Here's how the part is built. I have some questions about the finished solid (model axes, mm). Face numbers are marked on the shaded views. A direction names the side the tool comes from. Round coordinates to 2 decimals unless told otherwise and drop trailing zeros. Order: outer loops, then holes, each group sorted by start corner. A loop starts at its lowest first (then second) coordinate and runs counter-clockwise, first axis right, second up.
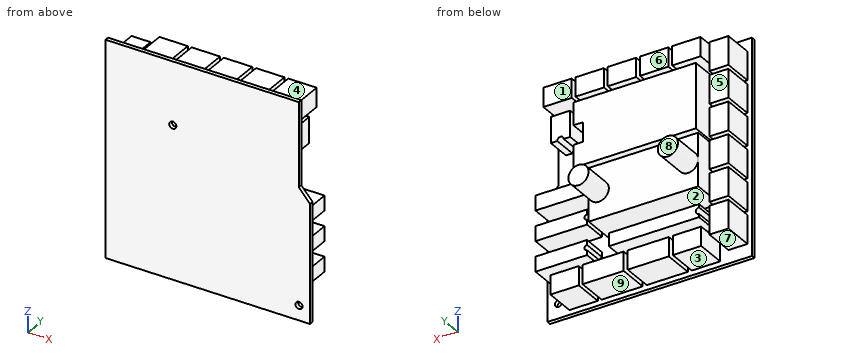
```python
from build123d import *

# Parameters (mm, degrees)
BOSS_EXTRUDE1_DEPTH = 1.5875
SKETCH2_R           = 1.3999972
CUT_EXTRUDE1_DEPTH  = 117.995510328
BOSS_EXTRUDE2_DEPTH = 11.90625
SKETCH4_W           = 43.17991364
SKETCH4_H           = 20.827958344
BOSS_EXTRUDE3_DEPTH = 13.49375
SKETCH6_R           = 3.96875
BOSS_EXTRUDE4_DEPTH = 12.7
BOSS_EXTRUDE5_DEPTH = 9.525


with BuildPart() as part:
    # Sketch1 → Boss-Extrude1 (new body)
    with BuildSketch(Plane(origin=(0, 0, 0), x_dir=(1, 0, 0), z_dir=(0, 1, 0))):
        Polygon((0.038099924, 84.724030552), (0.038099924, 0), (76.258247483, 0), (76.258247483, 33.070733858), (80.667638664, 38.11002378), (80.667638664, 84.724030552), align=None)
    extrude(amount=BOSS_EXTRUDE1_DEPTH)

    # Sketch2 → Cut-Extrude1 (cut, through all)
    with BuildSketch(Plane(origin=(0, 1.5875, 0), x_dir=(1, 0, 0), z_dir=(0, 1, 0))):
        with Locations(Location((76.336947326, 78.897342205, 0), (0, 0, 270))):
            Circle(SKETCH2_R)
        with Locations(Location((26.573446853, 24.724250551, 0), (0, 0, 270))):
            Circle(SKETCH2_R)
    extrude(amount=-CUT_EXTRUDE1_DEPTH, mode=Mode.SUBTRACT)

    # Sketch3 → Boss-Extrude2 (add)
    with BuildSketch(Plane(origin=(0, 1.5875, 0), x_dir=(1, 0, 0), z_dir=(0, 1, 0))):
        Polygon((60.822778354, 75.352649294), (60.822778354, 81.852636294), (60.822778354, 82.852634294), (72.022755954, 82.852634294), (72.022755954, 81.852636294), (72.022755954, 75.352649294), align=None)
        Polygon((59.322781354, 82.852634294), (59.322781354, 81.852636294), (59.322781354, 75.352649294), (43.122813754, 75.352649294), (43.122813754, 81.852636294), (43.122813754, 82.852634294), align=None)
        Polygon((25.342849314, 75.352649294), (25.342849314, 81.852636294), (25.342849314, 82.852634294), (41.542816914, 82.852634294), (41.542816914, 81.852636294), (41.542816914, 75.352649294), align=None)
        Polygon((63.597672804, 1.668196664), (63.597672804, 2.668194664), (63.597672804, 9.168181664), (74.797650404, 9.168181664), (74.797650404, 2.668194664), (74.797650404, 1.668196664), align=None)
        Polygon((50.897698204, 1.668196664), (50.897698204, 2.668194664), (50.897698204, 9.168181664), (62.097675804, 9.168181664), (62.097675804, 2.668194664), (62.097675804, 1.668196664), align=None)
        Polygon((38.197723604, 1.668196664), (38.197723604, 2.668194664), (38.197723604, 9.168181664), (49.397701204, 9.168181664), (49.397701204, 2.668194664), (49.397701204, 1.668196664), align=None)
        Polygon((36.697726604, 9.168181664), (36.697726604, 2.668194664), (36.697726604, 1.668196664), (25.497749004, 1.668196664), (25.497749004, 2.668194664), (25.497749004, 9.168181664), align=None)
        Polygon((12.797774404, 1.668196664), (12.797774404, 2.668194664), (12.797774404, 9.168181664), (23.997752004, 9.168181664), (23.997752004, 2.668194664), (23.997752004, 1.668196664), align=None)
        Polygon((9.318081364, 4.792990414), (2.818094364, 4.792990414), (1.818096364, 4.792990414), (1.818096364, 15.992968014), (2.818094364, 15.992968014), (9.318081364, 15.992968014), align=None)
        Polygon((1.818096364, 28.692942614), (2.818094364, 28.692942614), (9.318081364, 28.692942614), (9.318081364, 17.492965014), (2.818094364, 17.492965014), (1.818096364, 17.492965014), align=None)
        Polygon((9.318081364, 30.192939614), (2.818094364, 30.192939614), (1.818096364, 30.192939614), (1.818096364, 41.392917214), (2.818094364, 41.392917214), (9.318081364, 41.392917214), align=None)
        Polygon((9.318081364, 42.892914214), (2.818094364, 42.892914214), (1.818096364, 42.892914214), (1.818096364, 54.092891814), (2.818094364, 54.092891814), (9.318081364, 54.092891814), align=None)
        Polygon((1.818096364, 66.792866414), (2.818094364, 66.792866414), (9.318081364, 66.792866414), (9.318081364, 55.592888814), (2.818094364, 55.592888814), (1.818096364, 55.592888814), align=None)
        Polygon((12.562874874, 75.352649294), (12.562874874, 81.852636294), (12.562874874, 82.852634294), (23.762852474, 82.852634294), (23.762852474, 81.852636294), (23.762852474, 75.352649294), align=None)
        Polygon((1.818096364, 79.492841014), (2.818094364, 79.492841014), (9.318081364, 79.492841014), (9.318081364, 68.292863414), (2.818094364, 68.292863414), (1.818096364, 68.292863414), align=None)
    extrude(amount=BOSS_EXTRUDE2_DEPTH)

    # Sketch4 → Boss-Extrude3 (add)
    with BuildSketch(Plane(origin=(0, 1.5875, 0), x_dir=(1, 0, 0), z_dir=(0, 1, 0))):
        with Locations((34.317831364, 50.047999904)):
            Rectangle(SKETCH4_W, SKETCH4_H)
        Polygon((13.672772654, 17.343065314), (13.672772654, 32.583034834), (13.672772654, 37.663024674), (61.932676134, 37.663024674), (61.932676134, 28.773042454), (58.122683754, 28.773042454), (58.122683754, 21.153057694), (61.932676134, 21.153057694), (61.932676134, 12.263075474), (13.672772654, 12.263075474), align=None)
    extrude(amount=BOSS_EXTRUDE3_DEPTH)

    # Sketch6 → Boss-Extrude4 (add)
    with BuildSketch(Plane(origin=(0, 15.08125, 0), x_dir=(1, 0, 0), z_dir=(0, 1, 0))):
        with Locations(Location((16.696624544, 50.047999904, 0), (0, 0, 180))):
            Circle(SKETCH6_R)
        with Locations((51.939038184, 50.047999904)):
            Circle(SKETCH6_R)
    extrude(amount=BOSS_EXTRUDE4_DEPTH)

    # Sketch7 → Boss-Extrude5 (add)
    with BuildSketch(Plane(origin=(0, 1.5875, 0), x_dir=(1, 0, 0), z_dir=(0, 1, 0))):
        with BuildLine():
            Line((73.362653274, 22.423055154), (73.362653274, 12.263075474))
            Line((73.362653274, 12.263075474), (65.742668514, 12.263075474))
            Line((65.742668514, 12.263075474), (65.742668514, 22.423055154))
            Line((65.742668514, 22.423055154), (68.282663434, 22.423055154))
            ThreePointArc((68.282663434, 22.423055154), (69.552660894, 21.153057694), (70.822658354, 22.423055154))
            Line((70.822658354, 22.423055154), (73.362653274, 22.423055154))
        make_face()
        with BuildLine():
            Line((79.397641204, 46.710506579), (59.077681844, 46.710506579))
            Line((59.077681844, 46.710506579), (59.077681844, 44.805510389))
            ThreePointArc((59.077681844, 44.805510389), (60.093679812, 43.789512421), (59.077681844, 42.773514453))
            Line((59.077681844, 42.773514453), (59.077681844, 40.868518263))
            Line((59.077681844, 40.868518263), (79.397641204, 40.868518263))
            Line((79.397641204, 40.868518263), (79.397641204, 46.710506579))
        make_face()
        with BuildLine():
            Line((79.397641204, 58.587482825), (59.077681844, 58.587482825))
            Line((59.077681844, 58.587482825), (59.077681844, 56.682486635))
            ThreePointArc((59.077681844, 56.682486635), (60.093679812, 55.666488667), (59.077681844, 54.650490699))
            Line((59.077681844, 54.650490699), (59.077681844, 52.745494509))
            Line((59.077681844, 52.745494509), (79.397641204, 52.745494509))
            Line((79.397641204, 52.745494509), (79.397641204, 58.587482825))
        make_face()
        with BuildLine():
            Line((79.397641204, 70.423859152), (59.077681844, 70.423859152))
            Line((59.077681844, 70.423859152), (59.077681844, 68.518862962))
            ThreePointArc((59.077681844, 68.518862962), (60.093679812, 67.502864994), (59.077681844, 66.486867026))
            Line((59.077681844, 66.486867026), (59.077681844, 64.581870836))
            Line((59.077681844, 64.581870836), (79.397641204, 64.581870836))
            Line((79.397641204, 64.581870836), (79.397641204, 70.423859152))
        make_face()
        with BuildLine():
            Line((14.942770114, 65.917968164), (14.942770114, 64.647970704))
            Line((14.942770114, 64.647970704), (15.06976986, 64.647970704))
            Line((15.06976986, 64.647970704), (50.502698994, 64.647970704))
            Line((50.502698994, 64.647970704), (50.502698994, 69.727960544))
            Line((50.502698994, 69.727960544), (14.942770114, 69.727960544))
            Line((14.942770114, 69.727960544), (14.942770114, 68.457963084))
            ThreePointArc((14.942770114, 68.457963084), (16.212767574, 67.187965624), (14.942770114, 65.917968164))
        make_face()
    extrude(amount=BOSS_EXTRUDE5_DEPTH)


solid = part.part
```
1. If we section it at B-B, the plane z = -7.5: Write out the boundary of the cut face in (x, y).
Evaluation:
outline: (0.04, 0) - (76.26, 0) - (76.26, 1.59) - (74.8, 1.59) - (74.8, 13.49) - (63.6, 13.49) - (63.6, 1.59) - (62.1, 1.59) - (62.1, 13.49) - (50.9, 13.49) - (50.9, 1.59) - (49.4, 1.59) - (49.4, 13.49) - (38.2, 13.49) - (38.2, 1.59) - (36.7, 1.59) - (36.7, 13.49) - (25.5, 13.49) - (25.5, 1.59) - (24, 1.59) - (24, 13.49) - (12.8, 13.49) - (12.8, 1.59) - (9.32, 1.59) - (9.32, 13.49) - (1.82, 13.49) - (1.82, 1.59) - (0.04, 1.59) - close
2. If we mould it in two halves opening along Z, with no side actions, what happens to the marked faces 1, 2, 3 and 4? For each: released by +Z, released by -Z, zero draft, split by the parting line, or undercut.
Evaluation:
face 1: zero draft
face 2: undercut
face 3: released by -Z
face 4: released by +Z
3. If we section it at A-A, the plane x = 35: Write out the boundary of the cut face in (y, z), and give its area (3 significant figures).
Evaluation:
outline: (0, -84.72) - (1.59, -84.72) - (1.59, -82.85) - (13.49, -82.85) - (13.49, -75.35) - (1.59, -75.35) - (1.59, -69.73) - (11.11, -69.73) - (11.11, -64.65) - (1.59, -64.65) - (1.59, -60.46) - (15.08, -60.46) - (15.08, -39.63) - (1.59, -39.63) - (1.59, -37.66) - (15.08, -37.66) - (15.08, -12.26) - (1.59, -12.26) - (1.59, -9.17) - (13.49, -9.17) - (13.49, -1.67) - (1.59, -1.67) - (1.59, 0) - (0, 0) - close
area: 985 mm2
4. I need wall thicknesses on probe 1 along Z at (x, y) = (57, 5.25); probe 2 along Z at (x, y) = (21, 8.75); probe 3 along X at (y, z) = (8, -58.5). Which ranges of each line are inside material? Lowest first, please.
Evaluation:
probe 1: z = -82.85 to -75.35, -37.66 to -12.26, -9.17 to -1.67
probe 2: z = -82.85 to -75.35, -69.73 to -64.65, -60.46 to -39.63, -37.66 to -12.26, -9.17 to -1.67
probe 3: x = 1.82 to 9.32, 12.73 to 55.91, 59.08 to 79.4
5. On a 3-axis mill with a long thin cutter (end or side, diameter ignored), from which of +Z, -Z, +X, -X, +Y, -Y can I reach the whole of each face in a straight line? I mean the marked faces 5, 6, 7, 8 and 9. Say none if no direction works.
Evaluation:
face 5: +Z, -Z, -X, +Y
face 6: +Z, +X, -X, +Y
face 7: -Z, -X, +Y
face 8: +Z, -Z, +X, -X, +Y
face 9: -Z, +X, -X, +Y
6. If we section it at C-C, the plane y = 5.25: State how many separate pieces and enclosed holes the cut face has, and give its area (3 significant figures).
Evaluation:
separate pieces: 22
enclosed holes: 0
area: 4,040 mm2
7. If we section it at D-D, the plane y = 17.75: Write out the boundary of the cut face in (x, z).
Evaluation:
outline: circle Ø7.94 at (16.7, -50.05); circle Ø7.94 at (51.94, -50.05)
8. I'm going to push flat-ended pins straight in: P1, Ø3.5, axis at x = 7, y = 8, coming from the +Z side; P2, Ø2, axis at y = 8, z = -4, coming from the +X side; P3, Ø7.5, axis at x = 68.5, y = 7.5, coming from the +Z side. Where does each tip first touch, or does it pass through?
Evaluation:
P1: stops at z = -4.79
P2: stops at x = 74.8
P3: stops at z = -1.67
